For this review, take the finished solid that the model builds, in its own axes (mm). A direction names the side the tool comes from. Give positions to 0.01 mm unless a question says otherwise; leave off trailing zeros. Write each loop counter-clockwise with the first axis right and the second up, starting at its lowest first coordinate (ties: lowest second). Pieces come first, ordered by that corner, then holes. Notation, with made-up numbers: M 12.25,-7.5 L 62.25,-7.5 A22 cw 62.25,26.5 Z; hole C 58,14.5 d1. An arc over 180 degrees is marked long. One line per item, written item: value. Start each with the question number.
Item 1: Consider section A-A, the plane x = 38. Write out the cut boundary in (y, z).
Item 2: To check wall thickness, follow probe 1 along Z at (x, y) = (74, -2.25); probe 2 along Z at (x, y) = (155, -23); probe 3 along X at (y, z) = (-1.5, 8). State the ranges of each line that lie inside material, in increasing order.
Item 3: Tool access review of faces 1 (the face through (184.188, -13, -159)), 2 (the face through (93, -13, -127)), 3 (the face through (61, -13, 184.188)): name each direction out of +Z, -Z, +X, -X, +Y, -Y from which nothing blocks a thin tool from reaching the whole face with its end or side.
Item 4: Clearance check with flat-ended pins moving along their axes: pin 1 Ø7.5 at (x, y) = (96, -10.5) entering from -Z; pin 2 Ø2 at (x, y) = (-7.5, -10.5) entering from +Z; pin 3 Ø5 at (x, y) = (-30, -16.5) entering from -Z; pin 4 Ø1.5 at (x, z) = (-109.5, 69) entering from +Y. State where each tip first meets the part, or that it passes through.
Item 5: Consider section C-C, the plane x = 143. Write out the cut boundary in (y, z).
Item 6: Consider section D-D, the plane z = 0. Write out the cut boundary in (x, y), and give its area (3 significant figures).
Item 7: Consider section B-B, the plane y = -18.25. Write out the cut boundary in (x, z), and give its area (3 significant figures).
Item 8: Mouldability with a two-part tool opening along Y and no side actions: class faces 4 (the face through (59, -13, -184.188)), 5 (the face through (-3, 0, 130)), 6 (the face through (-3, -25.4, 130)) as released by +Y, released by -Y, zero draft, split by the parting line, or undercut.
```python
from build123d import *

# Parameters (mm, degrees)
F1_DEPTH = 25.4


with BuildPart() as f1:
    # F0 (on Front) → F1 (new body)
    with BuildSketch(Plane.XZ):
        with BuildLine():
            Line((120.687595, 184.187595), (0, 184.187595))
            ThreePointArc((0, 184.187595), (-184.187595, 0), (0, -184.187595))
            Line((0, -184.187595), (120.687595, -184.187595))
            Line((120.687595, -184.187595), (120.687595, -190.5))
            Line((120.687595, -190.5), (184.187595, -190.5))
            Line((184.187595, -190.5), (184.187595, -184.187595))
            Line((184.187595, -184.187595), (184.187595, -127))
            Line((184.187595, -127), (120.687595, -127))
            Line((120.687595, -127), (0, -127))
            ThreePointArc((0, -127), (-127, 0), (0, 127))
            Line((0, 127), (120.687595, 127))
            Line((120.687595, 127), (184.187595, 127))
            Line((184.187595, 127), (184.187595, 184.187595))
            Line((184.187595, 184.187595), (184.187595, 190.5))
            Line((184.187595, 190.5), (120.687595, 190.5))
            Line((120.687595, 190.5), (120.687595, 184.187595))
        make_face()
    extrude(amount=F1_DEPTH)


solid = f1.part
```
Model answer:
1. outline: M -25.4,-184.19 L 0,-184.19 L 0,-127 L -25.4,-127 Z; M -25.4,127 L 0,127 L 0,184.19 L -25.4,184.19 Z
2. probe 1: z = -184.19 to -127, 127 to 184.19
2. probe 2: z = -190.5 to -127, 127 to 190.5
2. probe 3: x = -184.01 to -126.75
3. face 1: +Z, -Z, +X, +Y, -Y
3. face 2: +X, +Y, -Y
3. face 3: +Z, -X, +Y, -Y
4. pin 1: stops at z = -184.19
4. pin 2: stops at z = 184.07
4. pin 3: stops at z = -182.12
4. pin 4: stops at y = 0
5. outline: M -25.4,-190.5 L 0,-190.5 L 0,-127 L -25.4,-127 Z; M -25.4,127 L 0,127 L 0,190.5 L -25.4,190.5 Z
6. outline: M -184.19,-25.4 L -127,-25.4 L -127,0 L -184.19,0 Z
6. area: 1,450 mm2
7. outline: M 0,-184.19 L 120.69,-184.19 L 120.69,-190.5 L 184.19,-190.5 L 184.19,-127 L 0,-127 A127 cw 0,127 L 184.19,127 L 184.19,190.5 L 120.69,190.5 L 120.69,184.19 L 0,184.19 A184.19 ccw Z
7. area: 49,800 mm2
8. face 4: zero draft
8. face 5: released by +Y
8. face 6: released by -Y
